Autodesk Inventor part; units mm, degrees
ref_plane "YZ Plane" through (0, 0, 0) normal (1, 0, 0) x (0, 1, 0)
ref_plane "XZ Plane" through (0, 0, 0) normal (0, 1, 0) x (-1, 0, 0)
ref_plane "XY Plane" through (0, 0, 0) normal (0, 0, 1) x (1, 0, 0)
sketch "Sketch1" plane through (0, 0, 0) normal (0, 0, 1) x (1, 0, 0)
  arc A0 (-10.9617, 7.0429) -> (7.0429, -10.9617) centre (6.25, 6.25) ccw
  arc A1 (-9.228, 7.7147) -> (-10.9617, 7.0429) centre (-9.9466, 6.9961) ccw
  line L0 (-4.9841, 3.4709) -> (-9.228, 7.7147)
  arc A2 (-4.054, 1.2253) -> (-4.9841, 3.4709) centre (-7.2298, 1.2253) ccw
  line L1 (-4.054, 0) -> (-4.054, 1.2253)
  arc A3 (-4.054, 0) -> (0, -4.054) centre (0, 0) ccw
  line L2 (1.2253, -4.054) -> (0, -4.054)
  arc A4 (3.4709, -4.9841) -> (1.2253, -4.054) centre (1.2253, -7.2298) ccw
  line L3 (7.7147, -9.228) -> (3.4709, -4.9841)
  arc A5 (7.0429, -10.9617) -> (7.7147, -9.228) centre (6.9961, -9.9466) ccw
  circle A6 centre (0, 0) radius 2.5
  arc A7 (5.2692, 3.756) -> (4.4, 1.6576) centre (7.3675, 1.6576) ccw
  line L4 (5.2692, 3.756) -> (8.6136, 7.1004)
  arc A8 (10.36, 6.377) -> (8.6136, 7.1004) centre (9.337, 6.377) ccw
  line L5 (10.36, 6.377) -> (10.36, 4.32)
  arc A9 (10.36, 4.32) -> (12.5, 4.32) centre (11.43, 4.32) ccw
  line L6 (12.5, 4.32) -> (12.5, 10.5209)
  arc A10 (12.5, 10.5209) -> (10.5209, 12.5) centre (10.5209, 10.5209) ccw
  line L7 (10.5209, 12.5) -> (4.32, 12.5)
  arc A11 (4.32, 12.5) -> (4.32, 10.36) centre (4.32, 11.43) ccw
  line L8 (4.32, 10.36) -> (6.377, 10.36)
  arc A12 (7.1004, 8.6136) -> (6.377, 10.36) centre (6.377, 9.337) ccw
  line L9 (7.1004, 8.6136) -> (3.6484, 5.1617)
  arc A13 (1.6576, 4.39) -> (3.6484, 5.1617) centre (1.6576, 7.344) ccw
  line L10 (1.6576, 4.39) -> (-1.6576, 4.39)
  arc A14 (-3.6484, 5.1617) -> (-1.6576, 4.39) centre (-1.6576, 7.344) ccw
  line L11 (-3.6484, 5.1617) -> (-7.1004, 8.6136)
  arc A15 (-6.377, 10.36) -> (-7.1004, 8.6136) centre (-6.377, 9.337) ccw
  line L12 (-6.377, 10.36) -> (-4.32, 10.36)
  arc A16 (-4.32, 10.36) -> (-4.32, 12.5) centre (-4.32, 11.43) ccw
  line L13 (-4.32, 12.5) -> (-10.5209, 12.5)
  arc A17 (-10.5209, 12.5) -> (-12.5, 10.5209) centre (-10.5209, 10.5209) ccw
  line L14 (-12.5, 10.5209) -> (-12.5, 6.25)
  arc A18 (-12.5, 6.25) -> (6.25, -12.5) centre (6.25, 6.25) ccw
  line L15 (6.25, -12.5) -> (10.5209, -12.5)
  arc A19 (10.5209, -12.5) -> (12.5, -10.5209) centre (10.5209, -10.5209) ccw
  line L16 (12.5, -10.5209) -> (12.5, -4.32)
  arc A20 (12.5, -4.32) -> (10.36, -4.32) centre (11.43, -4.32) ccw
  line L17 (10.36, -4.32) -> (10.36, -6.377)
  arc A21 (8.6136, -7.1004) -> (10.36, -6.377) centre (9.337, -6.377) ccw
  line L18 (8.6136, -7.1004) -> (5.2692, -3.756)
  arc A22 (4.4, -1.6576) -> (5.2692, -3.756) centre (7.3675, -1.6576) ccw
  line L19 (4.4, -1.6576) -> (4.4, 1.6576)
extrude "Extrusion1" add sketch "Sketch1" against normal blind 100
properties part number "25-2527-BLACK-FB"
Here's how the part is built. I have some questions about the finished solid (model axes, mm). A direction names the side the tool comes from. Give positions to 0.01 mm unless a question says otherwise; leave off trailing zeros. Loops run counter-clockwise (first coordinate to the right, second up) from the corner with the lowest first, then second, coordinate; pieces in that order, holes last. Notation, with made-up numbers: M 68.25,84.5 L 100.25,84.5 A10 ccw 100.25,102.5 Z; hole C 3.5,-35.5 d8. An arc over 180 degrees is marked long. Return JSON: item names as keys, results as strings.
Item 1: Imagine slicing it at C-C on z = -36.5. State how many separate pieces and enclosed holes the cut face has, then the cut area to 3 significant figures.
A:
{"separate pieces": "1", "enclosed holes": "2", "area": "240 mm^2"}
Item 2: Please list where these lines run through material, in increasing order: line 1 (Y direction, x = 0, z = -70); line 2 (Y direction, x = 6.5, z = -69.5); line 3 (X direction, y = -6.5, z = -52.5).
A:
{"line 1": "y = -11.43 to -9.81, -4.05 to -2.5, 2.5 to 4.39", "line 2": "y = -12.5 to -10.98, -8.01 to -4.99, 4.99 to 8.01, 10.35 to 12.5", "line 3": "x = -7.5 to -5.34, 4.99 to 8.01, 10.35 to 12.5"}
Item 3: On a 3-axis mill with a long thin cutter (end or side, diameter ignored), from which of +Z, -Z, +X, -X, +Y, -Y can I reach the whole of each face in a straight line? I mean faces 4 (the flat face through (4.4, 0, -49)), 5 (the cylindrical face through (-3.25, 11.41, -49.3)), 6 (the flat face through (0, 3, -100)). Say none if no direction works.
A:
{"face 4": "+Z, -Z, +X", "face 5": "+Z, -Z", "face 6": "-Z, +X, -X, +Y, -Y"}
Item 4: Thinking about a two-plate mould opening in Y: for faces 1 (the flat face through (-7, 12.5, -49)), 2 (the cylindrical face through (11.9, -11.94, -49.3)), 3 (the cylindrical face through (11.41, 3.25, -49.3)), which applies, released by +Y, released by -Y, zero draft, split by the parting line, or undercut?
A:
{"face 1": "released by +Y", "face 2": "released by -Y", "face 3": "undercut"}
Item 5: I'm going to push flat-ended pins straight in: pin 1 Ø3 at (x, z) = (0.5, -66.5) entering from -Y; pin 2 Ø3.5 at (y, z) = (-0.5, -45.5) entering from +X; pin 3 Ø1 at (x, z) = (5.5, -33) entering from -Y; pin 4 Ø1 at (x, y) = (-3, -3.5) entering from -Z. Where does each tip first touch, or does it pass through?
A:
{"pin 1": "stops at y = -12.01", "pin 2": "stops at x = 4.46", "pin 3": "stops at y = -12.5", "pin 4": "passes through"}
Item 6: Imagine slicing it at A-A on x = 11.43. List the corners of the cut face in (y, z) for me.
A:
{"outline": "M -12.28,-100 L -3.25,-100 L -3.25,0 L -12.28,0 Z; M 3.25,-100 L 12.28,-100 L 12.28,0 L 3.25,0 Z"}
